Input: dimensioned drawing with shaded views. Units: mm. Origin: part minimum x, y, z. Give positions to 0.01 mm unless a question says otherwise; leave off trailing zeros. Order: outer loops, then holes, each group sorted by start corner. A loop starts at its lowest first (then second) coordinate and runs counter-clockwise, first axis right, second up. Notation, with made-up numbers: (67, 21) - (125, 21) arc R28 cw to (125, 44) - close; hole circle Ø11 at (-5, 39). An arc over 180 degrees is marked (long way). Answer as CSV lines item,"result".
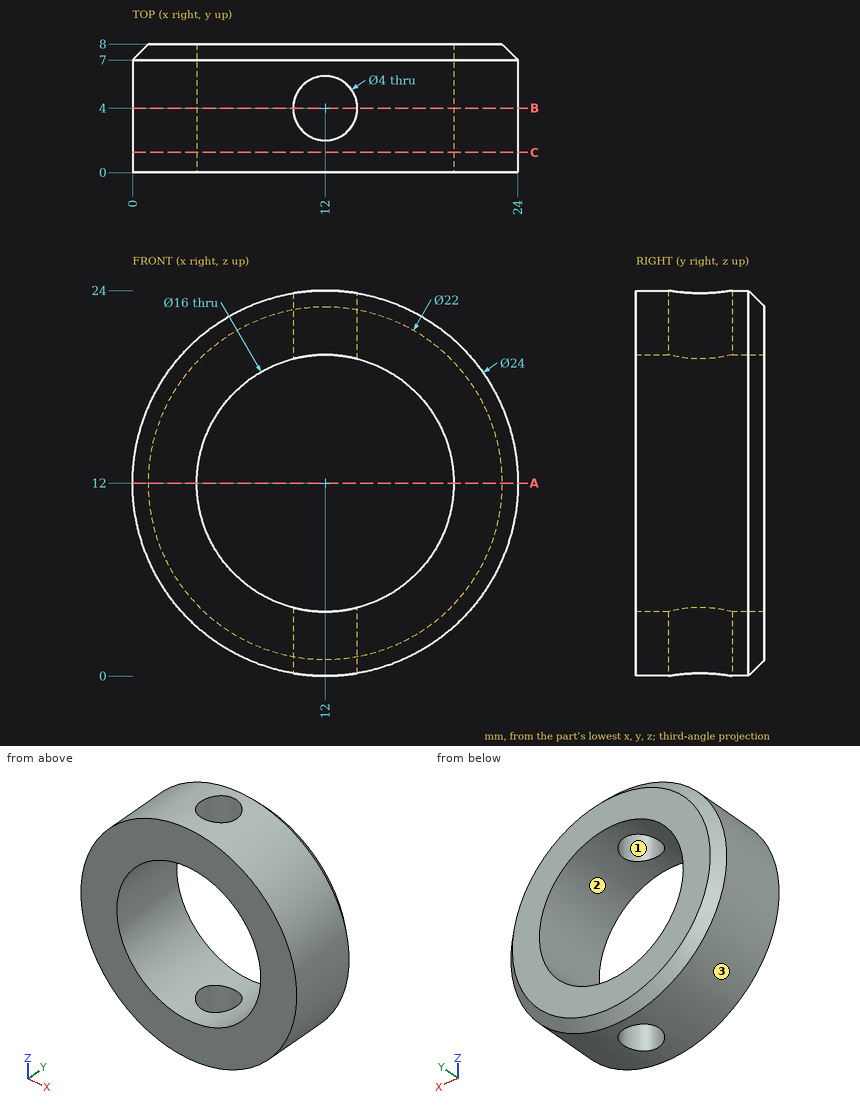
(1) Cut plane B-B (y = 4). Return loops of the section in (x, z), then the cut area to 3 significant figures.
Completed:
outline,"(10, 0.17) - (10, 4.25) arc R8 cw to (10, 19.75) - (10, 23.83) arc R12 ccw to start; (14, 0.17) arc R12 ccw to (14, 23.83) - (14, 19.75) arc R8 cw to (14, 4.25) - close"
area,"219 mm²"
(2) Cut plane A-A (z = 12). Return loops of the section in (x, y).
Completed:
outline,"(0, 0) - (4, 0) - (4, 8) - (1, 8) - (0, 7) - close; (20, 0) - (24, 0) - (24, 7) - (23, 8) - (20, 8) - close"
(3) Ray query, line 1 (X direction, y = 4, z = 12); line 2 (X direction, y = 7.75, z = 10); line 3 (Z direction, x = 11, y = 1). Return the intervals inside material, ascending. Write a range as from..to.
Completed:
line 1,"0..4, 20..24"
line 2,"0.93..4.25, 19.75..23.07"
line 3,"0.04..4.06, 19.94..23.96"
(4) Mould query, pull axis Z, two halves, no side actions, for the marked faces 1, 2 and 3. Classes: released by +Z, released by -Z, zero draft, split by the parting line, or undercut.
Completed:
face 1,"zero draft"
face 2,"undercut"
face 3,"split by the parting line"
(5) Contact query for a flat-ended pin moving along its axis: pin 1 (1 mm diameter, centred on x = 5.5, y = 5.5, fed in from -Z). Output: stop coordinate, or through.
Completed:
pin 1,"z = 1.61"
(6) Cut plane C-C (y = 1.25). Return loops of the section in (x, z).
Completed:
outline,"circle Ø24 at (12, 12); hole circle Ø16 at (12, 12)"
